Source: CAD feature listing. Evaluate the final solid. Frame: model axes, mm. A direction names the side the tool comes from. Give positions to 0.01 mm unless a question says otherwise; leave off trailing zeros. Loops run counter-clockwise (first coordinate to the right, second up) from the corner with the lowest first, then second, coordinate; pieces in that order, holes last.
```python
from build123d import *

# Parameters (mm, degrees)
BOSS_EXTRUDE1_DEPTH = 3
SKETCH2_W           = 13
SKETCH2_H           = 22.7
SKETCH2_W_2         = 6.499
SKETCH2_H_2         = 2.399
CUT_EXTRUDE1_DEPTH  = 3


with BuildPart() as part:
    # Sketch1 → Boss-Extrude1 (new body)
    with BuildSketch(Plane.XY):
        with BuildLine():
            ThreePointArc((-27.048045715, 1.346978667), (-23.229413898, -7.644456097), (-16.294351646, -14.524336884))
            ThreePointArc((-16.294351646, -14.524336884), (-14.971129192, -15.233831637), (-13.702557421, -16.036966825))
            ThreePointArc((-13.702557421, -16.036966825), (-7.036411487, -18.317683791), (0, -18.675573281))
            ThreePointArc((0, -18.675573281), (7.036411487, -18.317683791), (13.702557421, -16.036966825))
            ThreePointArc((13.702557421, -16.036966825), (14.971129192, -15.233831637), (16.294351646, -14.524336884))
            ThreePointArc((16.294351646, -14.524336884), (23.229413898, -7.644456097), (27.048045715, 1.346978667))
            ThreePointArc((27.048045715, 1.346978667), (22.641390956, 7.722324922), (16.597159635, 12.573192245))
            ThreePointArc((16.597159635, 12.573192245), (16.261784348, 12.757647773), (15.931841919, 12.951654004))
            ThreePointArc((15.931841919, 12.951654004), (8.210400332, 15.763932748), (0, 16.108749071))
            ThreePointArc((0, 16.108749071), (-8.210400332, 15.763932748), (-15.931841919, 12.951654004))
            ThreePointArc((-15.931841919, 12.951654004), (-16.261784348, 12.757647773), (-16.597159635, 12.573192245))
            ThreePointArc((-16.597159635, 12.573192245), (-22.641390956, 7.722324922), (-27.048045715, 1.346978667))
        make_face()
        with BuildLine():
            Line((29.524, 9.802), (29.524, -9.802))
            Line((29.524, -9.802), (32.624, -9.802))
            Line((32.624, -9.802), (32.624, -12.802))
            Line((32.624, -12.802), (34.17489845, -12.539239659))
            ThreePointArc((34.17489845, -12.539239659), (38.013587392, 0.074463168), (34.262667869, 12.714543648))
            Line((34.262667869, 12.714543648), (32.624, 12.802))
            Line((32.624, 12.802), (32.624, 9.802))
            Line((32.624, 9.802), (29.524, 9.802))
        make_face()
        with BuildLine():
            ThreePointArc((27.048045715, 1.346978667), (23.229413898, -7.644456097), (16.294351646, -14.524336884))
            ThreePointArc((16.294351646, -14.524336884), (22.767282146, -12.573251909), (29.524, -12.802))
            Line((29.524, -12.802), (29.524, -9.802))
            Line((29.524, -9.802), (29.524, 9.802))
            Line((29.524, 9.802), (29.524, 12.802))
            ThreePointArc((29.524, 12.802), (23.09016911, 11.015904248), (16.597159635, 12.573192245))
            ThreePointArc((16.597159635, 12.573192245), (22.641390956, 7.722324922), (27.048045715, 1.346978667))
        make_face()
        with BuildLine():
            Line((-29.524, -9.802), (-29.524, -12.802))
            ThreePointArc((-29.524, -12.802), (-22.767282146, -12.573251909), (-16.294351646, -14.524336884))
            ThreePointArc((-16.294351646, -14.524336884), (-23.229413898, -7.644456097), (-27.048045715, 1.346978667))
            ThreePointArc((-27.048045715, 1.346978667), (-22.641390956, 7.722324922), (-16.597159635, 12.573192245))
            ThreePointArc((-16.597159635, 12.573192245), (-23.09016911, 11.015904248), (-29.524, 12.802))
            Line((-29.524, 12.802), (-29.524, 9.802))
            Line((-29.524, 9.802), (-29.524, -9.802))
        make_face()
        with BuildLine():
            Line((-32.624, -9.802), (-29.524, -9.802))
            Line((-29.524, -9.802), (-29.524, 9.802))
            Line((-29.524, 9.802), (-32.624, 9.802))
            Line((-32.624, 9.802), (-32.624, 12.802))
            Line((-32.624, 12.802), (-34.262667869, 12.714543648))
            ThreePointArc((-34.262667869, 12.714543648), (-38.013587392, 0.074463168), (-34.17489845, -12.539239659))
            Line((-34.17489845, -12.539239659), (-32.624, -12.802))
            Line((-32.624, -12.802), (-32.624, -9.802))
        make_face()
    extrude(amount=-BOSS_EXTRUDE1_DEPTH)

    # Sketch2 → Cut-Extrude1 (cut)
    with BuildSketch(Plane.XY):
        with BuildLine():
            ThreePointArc((-18.140073475, 1.691900685), (-18.886998155, 1.858903562), (-19.297064795, 2.505147934))
            Line((-19.297064795, 2.505147934), (-19.762150522, 5.170880716))
            ThreePointArc((-19.762150522, 5.170880716), (-19.595147646, 5.917805396), (-18.948903274, 6.327872035))
            Line((-18.948903274, 6.327872035), (-11.398949082, 7.645099315))
            ThreePointArc((-11.398949082, 7.645099315), (-10.652024403, 7.478096438), (-10.241957763, 6.831852066))
            Line((-10.241957763, 6.831852066), (-9.776872035, 4.166119284))
            ThreePointArc((-9.776872035, 4.166119284), (-9.943874912, 3.419194604), (-10.590119284, 3.009127965))
            Line((-10.590119284, 3.009127965), (-18.140073475, 1.691900685))
        make_face()
        Rectangle(SKETCH2_W, SKETCH2_H)
        with BuildLine():
            ThreePointArc((-16.351, -9.502), (-17.058106781, -9.209106781), (-17.351, -8.502))
            Line((-17.351, -8.502), (-17.351, -2.991))
            ThreePointArc((-17.351, -2.991), (-17.058106781, -2.283893219), (-16.351, -1.991))
            Line((-16.351, -1.991), (-9.605, -1.991))
            ThreePointArc((-9.605, -1.991), (-8.897893219, -2.283893219), (-8.605, -2.991))
            Line((-8.605, -2.991), (-8.605, -8.502))
            ThreePointArc((-8.605, -8.502), (-8.897893219, -9.209106781), (-9.605, -9.502))
            Line((-9.605, -9.502), (-16.351, -9.502))
        make_face()
        with BuildLine():
            Line((9.605, -1.991), (16.351, -1.991))
            ThreePointArc((16.351, -1.991), (17.058106781, -2.283893219), (17.351, -2.991))
            Line((17.351, -2.991), (17.351, -8.502))
            ThreePointArc((17.351, -8.502), (17.058106781, -9.209106781), (16.351, -9.502))
            Line((16.351, -9.502), (9.605, -9.502))
            ThreePointArc((9.605, -9.502), (8.897893219, -9.209106781), (8.605, -8.502))
            Line((8.605, -8.502), (8.605, -2.991))
            ThreePointArc((8.605, -2.991), (8.897893219, -2.283893219), (9.605, -1.991))
        make_face()
        with BuildLine():
            ThreePointArc((10.241957763, 6.831852066), (10.652024403, 7.478096438), (11.398949082, 7.645099315))
            Line((11.398949082, 7.645099315), (18.948903274, 6.327872035))
            ThreePointArc((18.948903274, 6.327872035), (19.595147646, 5.917805396), (19.762150522, 5.170880716))
            Line((19.762150522, 5.170880716), (19.297064795, 2.505147934))
            ThreePointArc((19.297064795, 2.505147934), (18.886998155, 1.858903562), (18.140073475, 1.691900685))
            Line((18.140073475, 1.691900685), (10.590119284, 3.009127965))
            ThreePointArc((10.590119284, 3.009127965), (9.943874912, 3.419194604), (9.776872035, 4.166119284))
            Line((9.776872035, 4.166119284), (10.241957763, 6.831852066))
        make_face()
        with Locations((0, -16.3075)):
            Rectangle(SKETCH2_W_2, SKETCH2_H_2)
    extrude(amount=-CUT_EXTRUDE1_DEPTH, mode=Mode.SUBTRACT)


solid = part.part
```
(1) Section D-D, the plane x = 7.5. Return the cut outline in (y, z).
A:
outline: (-18.22, -3) - (15.89, -3) - (15.89, 0) - (-18.22, 0) - close
(2) Ray query, line 1 along Y through (x, z) = (-11, -2.1); line 2 along Y through (x, z) = (14, -1.9); line 3 along X through (y, z) = (-0.5, -2.55). Return the intervals inside material, ascending.
A:
line 1: y = -17.21 to -9.5, -1.99 to 2.94, 7.63 to 15.05
line 2: y = -15.84 to -9.5, -1.99 to 2.41, 7.19 to 13.92
line 3: x = -38 to -6.5, 6.5 to 38
(3) First-contact query: pin 1 (1.5 mm diameter, centred on y = -7, z = -1.5, fed in from +X); pin 2 (0.9 mm diameter, centred on y = 11.5, z = -1, fed in from -X); pin 3 (1.5 mm diameter, centred on x = -31, z = -1.5, fed in from -Y). Flat tips, straight axial feed; report the tip coordinate or a pass-through.
A:
pin 1: stops at x = 37.1
pin 2: stops at x = -35.26
pin 3: stops at y = -9.8
(4) Section C-C, the plane z = -2.45. Count the separate pieces of the cut face and the enclosed holes in it, then the cut area to 3 significant figures.
A:
separate pieces: 1
enclosed holes: 6
area: 1,520 mm2
(5) Section A-A, the plane x = -15. Return the cut outline in (y, z).
A:
outline: (-15.22, -3) - (-9.5, -3) - (-9.5, 0) - (-15.22, 0) - close; (-1.99, -3) - (2.24, -3) - (2.24, 0) - (-1.99, 0) - close; (7.02, -3) - (13.44, -3) - (13.44, 0) - (7.02, 0) - close
(6) Reachability of faces 3 (the flat face through (-29.524, 11, -1)), 4 (the cylindrical face through (38.012, -0.113, -1.479)), 5 (the flat face through (-32.624, -11, -1)), 6 (the flat face through (13, -9.502, -1)) from +Z, -Z, +X, -X, +Y, -Y: full face, straight path, thin tool, end or side. Return the list, or none.
A:
face 3: +Z, -Z, +Y
face 4: +Z, -Z, +X
face 5: +Z, -Z, -Y
face 6: +Z, -Z
(7) Section B-B, the plane x = 31. Return the cut outline in (y, z), then the cut area to 3 significant figures.
A:
outline: (-9.8, -3) - (9.8, -3) - (9.8, 0) - (-9.8, 0) - close
area: 58.8 mm2
(8) Mould query, pull axis X, two halves, no side actions, for faces 1 (the flat face through (33.455, 12.758, -1.479)), 2 (the flat face through (-19.526, 3.819, -1.479)). Classes: pulls with the +X half, pulls with the -X half, needs draft (parallel to the pull), parting line crosses it, or undercut.
A:
face 1: pulls with the +X half
face 2: undercut
